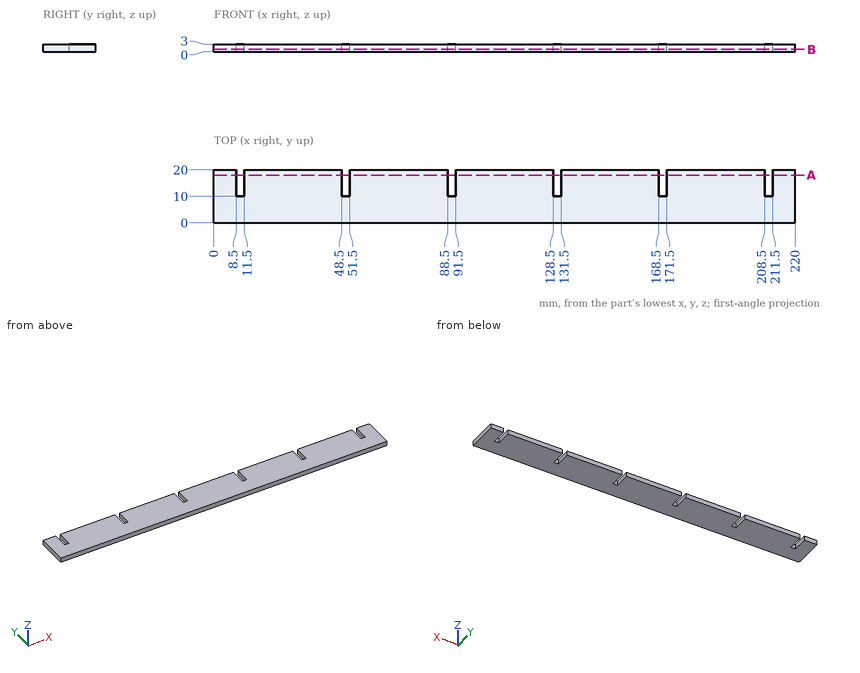
Job drawing, mm, ordinate dimensions from the low corner. One solid piece. Round coordinates to 2 decimals unless told otherwise and drop trailing zeros. Order: outer loops, then holes, each group sorted by start corner. A loop starts at its lowest first (then second) coordinate and runs counter-clockwise, first axis right, second up. Notation, with made-up numbers: (-24.5, 53) -> (0.5, 53) arc R13 ccw to (0.5, 59) -> close; hole circle Ø1 at (65.25, 73). An arc over 180 degrees is marked (long way). Write item = value, one per line.
(1) Drill centre line: L1, parallel to Y at x = 10, z = 0.25. Where is it in solid material? Low to high.
Answers follow:
L1 = 0 to 10
(2) Cut at B-B (z = 1). Write the cut outline in (x, y), plus the area to 3 significant figures.
Answers follow:
outline = (0, 0) -> (220, 0) -> (220, 20) -> (211.5, 20) -> (211.5, 10) -> (208.5, 10) -> (208.5, 20) -> (171.5, 20) -> (171.5, 10) -> (168.5, 10) -> (168.5, 20) -> (131.5, 20) -> (131.5, 10) -> (128.5, 10) -> (128.5, 20) -> (91.5, 20) -> (91.5, 10) -> (88.5, 10) -> (88.5, 20) -> (51.5, 20) -> (51.5, 10) -> (48.5, 10) -> (48.5, 20) -> (11.5, 20) -> (11.5, 10) -> (8.5, 10) -> (8.5, 20) -> (0, 20) -> close
area = 4,220 mm²
(3) Cut at A-A (y = 18). Write the cut outline in (x, z).
Answers follow:
outline = (0, 0) -> (8.5, 0) -> (8.5, 3) -> (0, 3) -> close; (11.5, 0) -> (48.5, 0) -> (48.5, 3) -> (11.5, 3) -> close; (51.5, 0) -> (88.5, 0) -> (88.5, 3) -> (51.5, 3) -> close; (91.5, 0) -> (128.5, 0) -> (128.5, 3) -> (91.5, 3) -> close; (131.5, 0) -> (168.5, 0) -> (168.5, 3) -> (131.5, 3) -> close; (171.5, 0) -> (208.5, 0) -> (208.5, 3) -> (171.5, 3) -> close; (211.5, 0) -> (220, 0) -> (220, 3) -> (211.5, 3) -> close
(4) Flat gauge pin, fed straight in: P1, Ø1.5, axis at x = 90.5, z = 1, coming from the +Y side. Where does the tip first touch, or does it go through?
Answers follow:
P1 = 10
